CAD build for the part. Positions are in the model's coordinates, mm. Coordinates: 2 decimals unless noted, no trailing zeros. Order: outer loops, then holes, each group sorted by start corner. A loop starts at its lowest first (then second) coordinate and runs counter-clockwise, first axis right, second up. Notation, with made-up numbers: (56.25, 17) - (86.25, 17) arc R18 ccw to (86.25, 40) - close; hole circle Ø1 at (86.5, 40.5). An arc over 180 degrees is marked (long way). Use one line per item in the form item = value.
```python
from build123d import *
from OCP.BRepFilletAPI import BRepFilletAPI_MakeChamfer

# Parameters (mm, degrees)
SKETCH1_W             = 60
SKETCH1_H             = 180
BOSS_EXTRUDE1_DEPTH   = 6
CHAMFER2_SIZE         = 10
BOSS_EXTRUDE3_DEPTH   = 6
BOSS_EXTRUDE4_DEPTH   = 6
CHAMFER14_SIZE        = 2
CHAMFER16_SIZE        = 7
CHAMFER16_SIZE2       = 56.79198309
CHAMFER17_SIZE        = 2
SKETCH59_W            = 21.7
SKETCH59_H            = 5
BOSS_EXTRUDE5_DEPTH   = 6
CHAMFER19_SIZE        = 5
CUT_EXTRUDE28_DEPTH   = 112.04216162
CHAMFER20_SIZE        = 3
CHAMFER20_SIZE2       = 3.484649721
CUT_EXTRUDE29_DEPTH   = 111.166083192
CHAMFER24_SIZE        = 1
CUT_EXTRUDE31_DEPTH   = 111.166083332
SKETCH66_R            = 6
BOSS_EXTRUDE6_DEPTH   = 6
BOSS_EXTRUDE7_DEPTH   = 6
BOSS_EXTRUDE8_DEPTH   = 6
BOSS_EXTRUDE9_DEPTH   = 6
F_3_0MM_DOWEL_HOLE3_D = 3.5


with BuildPart() as part:
    # Sketch1 → Boss-Extrude1 (new body)
    with BuildSketch(Plane(origin=(0, 0, 0), x_dir=(1, 0, 0), z_dir=(0, 1, 0))):
        Rectangle(SKETCH1_W, SKETCH1_H)
    extrude(amount=BOSS_EXTRUDE1_DEPTH)

    # Chamfer2
    chamfer2_edges = [part.edges().sort_by_distance(p)[0] for p in [
        (-30, 3, -90),
        (30, 3, -90),
        (30, 3, 90),
        (-30, 3, 90),
    ]]
    chamfer(chamfer2_edges, length=CHAMFER2_SIZE)

    # Sketch52 → Boss-Extrude3 (add, through all)
    with BuildSketch(Plane(origin=(0, 6, 0), x_dir=(1, 0, 0), z_dir=(0, 1, 0))):
        Polygon((45, 53.067924807), (36.85, 44.173760523), (30, 25.3535402), (30, 79.656998575), (33.429823026, 66.856724783), align=None)
        Polygon((-33.429823026, 66.856724783), (-45, 53.067924807), (-36.85, 44.173760523), (-30, 25.3535402), (-30, 79.656998575), align=None)
    extrude(amount=-BOSS_EXTRUDE3_DEPTH)

    # Sketch53 → Boss-Extrude4 (add, through all)
    with BuildSketch(Plane(origin=(0, 6, 0), x_dir=(1, 0, 0), z_dir=(0, 1, 0))):
        Polygon((30, -65.989627063), (30, -80), (39, -98.344262241), (51.212964584, -83.789417822), align=None)
        Polygon((-51.212964584, -83.789417822), (-30, -65.989627063), (-30, -80), (-39, -98.344262241), align=None)
    extrude(amount=-BOSS_EXTRUDE4_DEPTH)

    # Chamfer14
    chamfer14_edges = [part.edges().sort_by_distance(p)[0] for p in [
        (-45.106482292, 6, 91.066840031),
        (45.106482292, 6, 91.066840031),
    ]]
    chamfer(chamfer14_edges, length=CHAMFER14_SIZE)

    # Chamfer16: one chamfer whose edges measure the first distance from different faces: ONE call of the kernel's chamfer builder (chamfer() names one face for all edges)
    chamfer16_edges_1 = [part.edges().sort_by_distance(p)[0] for p in [
        (-30, 3, 65.989627063),
    ]]
    chamfer16_side_1 = [part.faces().sort_by_distance(p)[0] for p in [
        (-40.483474971, 2.971570606, 74.786307045),
    ]]
    chamfer16_edges_2 = [part.edges().sort_by_distance(p)[0] for p in [
        (30, 3, 65.989627063),
    ]]
    chamfer16_side_2 = [part.faces().sort_by_distance(p)[0] for p in [
        (40.483474971, 2.971570606, 74.786307045),
    ]]
    chamfer16 = BRepFilletAPI_MakeChamfer(part.part.solid().wrapped)
    for e in chamfer16_edges_1:
        chamfer16.Add(CHAMFER16_SIZE, CHAMFER16_SIZE2, e.wrapped, chamfer16_side_1[0].wrapped)  # the first distance lies on this face
    for e in chamfer16_edges_2:
        chamfer16.Add(CHAMFER16_SIZE, CHAMFER16_SIZE2, e.wrapped, chamfer16_side_2[0].wrapped)  # the first distance lies on this face
    add(Compound.cast(chamfer16.Shape()), mode=Mode.REPLACE)

    # Chamfer17
    chamfer17_edges = [part.edges().sort_by_distance(p)[0] for p in [
        (39.214911513, 6, -59.962324795),
        (-39.214911513, 6, -59.962324795),
    ]]
    chamfer(chamfer17_edges, length=CHAMFER17_SIZE)

    # Sketch59 → Boss-Extrude5 (add, through all)
    with BuildSketch(Plane(origin=(0, 6, 0), x_dir=(1, 0, 0), z_dir=(0, 1, 0))):
        with Locations((0, -92.5)):
            Rectangle(SKETCH59_W, SKETCH59_H)
    extrude(amount=-BOSS_EXTRUDE5_DEPTH)

    # Chamfer19
    chamfer19_edges = [part.edges().sort_by_distance(p)[0] for p in [
        (0, 0, 95),
    ]]
    chamfer(chamfer19_edges, length=CHAMFER19_SIZE)

    # Sketch61 → Cut-Extrude28 (cut, through all)
    with BuildSketch(Plane.XZ):
        Polygon((30, -79.656998575), (20, -90), (30, -80), align=None)
        Polygon((-30, -80), (-30, -79.656998575), (-20, -90), align=None)
    extrude(amount=-CUT_EXTRUDE28_DEPTH, mode=Mode.SUBTRACT)

    # Chamfer20: one chamfer whose edges measure the first distance from different faces: ONE call of the kernel's chamfer builder (chamfer() names one face for all edges)
    chamfer20_edges_1 = [part.edges().sort_by_distance(p)[0] for p in [
        (-45, 2, -53.067924807),
    ]]
    chamfer20_side_1 = [part.faces().sort_by_distance(p)[0] for p in [
        (-40.821197815, 2.933105821, -48.507562458),
    ]]
    chamfer20_edges_2 = [part.edges().sort_by_distance(p)[0] for p in [
        (45, 2, -53.067924807),
    ]]
    chamfer20_side_2 = [part.faces().sort_by_distance(p)[0] for p in [
        (39.214911513, 2, -59.962324795),
    ]]
    chamfer20_edges_3 = [part.edges().sort_by_distance(p)[0] for p in [
        (-51.212964584, 2, 83.789417822),
        (51.212964584, 2, 83.789417822),
    ]]
    chamfer20 = BRepFilletAPI_MakeChamfer(part.part.solid().wrapped)
    for e in chamfer20_edges_1:
        chamfer20.Add(CHAMFER20_SIZE, CHAMFER20_SIZE2, e.wrapped, chamfer20_side_1[0].wrapped)  # the first distance lies on this face
    for e in chamfer20_edges_2:
        chamfer20.Add(CHAMFER20_SIZE, CHAMFER20_SIZE2, e.wrapped, chamfer20_side_2[0].wrapped)  # the first distance lies on this face
    for e in chamfer20_edges_3:
        chamfer20.Add(CHAMFER20_SIZE, e.wrapped)
    add(Compound.cast(chamfer20.Shape()), mode=Mode.REPLACE)

    # Sketch62 → Cut-Extrude29 (cut, through all)
    with BuildSketch(Plane(origin=(0, 6, 0), x_dir=(1, 0, 0), z_dir=(0, 1, 0))):
        with BuildLine():
            Line((20, 90), (30, 79.656998575))
            Line((30, 79.656998575), (33.429823026, 66.856724783))
            add(Edge.make_bspline(
                [(33.429823026, 66.856724783), (13.849706238, 74.804707739), (20, 74.573823319), (20, 90)],
                knots=[0, 0, 0, 0, 1, 1, 1, 1], degree=3))
        make_face()
        with BuildLine():
            Line((-30, 79.656998575), (-33.429823026, 66.856724783))
            add(Edge.make_bspline(
                [(-33.429823026, 66.856724783), (-13.849706238, 74.804707739), (-20, 74.573823319), (-20, 90)],
                knots=[0, 0, 0, 0, 1, 1, 1, 1], degree=3))
            Line((-20, 90), (-30, 79.656998575))
        make_face()
    extrude(amount=-CUT_EXTRUDE29_DEPTH, mode=Mode.SUBTRACT)

    # Chamfer24
    chamfer24_edges = [part.edges().sort_by_distance(p)[0] for p in [
        (0, 0, -90),
    ]]
    chamfer(chamfer24_edges, length=CHAMFER24_SIZE)

    # Sketch64 → Cut-Extrude31 (cut, through all)
    with BuildSketch(Plane(origin=(0, 6, 0), x_dir=(1, 0, 0), z_dir=(0, 1, 0))):
        with BuildLine():
            Line((36.85, 44.173760523), (25, 5.3535402))
            add(Edge.make_bspline(
                [(25, 5.3535402), (25, 11.888533403), (26.675205792, 28.424746849), (35.495075594, 42.695120001), (36.85, 44.173760523)],
                knots=[0, 0, 0, 0, 0.750989917, 1, 1, 1, 1], degree=3))
        make_face()
        with BuildLine():
            Line((-36.85, 44.173760523), (-25, 5.3535402))
            add(Edge.make_bspline(
                [(-25, 5.3535402), (-25, 11.888533403), (-26.675205792, 28.424746849), (-35.495075594, 42.695120001), (-36.85, 44.173760523)],
                knots=[0, 0, 0, 0, 0.750989917, 1, 1, 1, 1], degree=3))
        make_face()
    extrude(amount=-CUT_EXTRUDE31_DEPTH, mode=Mode.SUBTRACT)

    # Sketch66 → Boss-Extrude6 (add)
    with BuildSketch(Plane(origin=(0, 6, 0), x_dir=(1, 0, 0), z_dir=(0, 1, 0))):
        with Locations((29.320888862, -18)):
            Circle(SKETCH66_R)
        with BuildLine():
            ThreePointArc((25, -13.837078017), (26.973287097, -12.478336668), (29.320888862, -12))
            Line((29.320888862, -12), (25, -12))
            Line((25, -12), (25, -13.837078017))
        make_face()
        with BuildLine():
            Line((25, -24), (29.320888862, -24))
            ThreePointArc((29.320888862, -24), (26.973287097, -23.521663332), (25, -22.162921983))
            Line((25, -22.162921983), (25, -24))
        make_face()
        with Locations((-29.320888862, -18)):
            Circle(SKETCH66_R)
        with BuildLine():
            Line((-25, -12), (-29.320888862, -12))
            ThreePointArc((-29.320888862, -12), (-26.973287097, -12.478336668), (-25, -13.837078017))
            Line((-25, -13.837078017), (-25, -12))
        make_face()
        with BuildLine():
            ThreePointArc((-25, -22.162921983), (-26.973287097, -23.521663332), (-29.320888862, -24))
            Line((-29.320888862, -24), (-25, -24))
            Line((-25, -24), (-25, -22.162921983))
        make_face()
    extrude(amount=-BOSS_EXTRUDE6_DEPTH)

    # Sketch67 → Boss-Extrude7 (add)
    with BuildSketch(Plane.XZ):
        with BuildLine():
            Line((30, -21.733379998), (30, -31.878802778))
            add(Edge.make_bspline(
                [(30, -31.878802778), (26.006043433, -21.746256389), (25, -11.197434735), (25, -5.3535402)],
                knots=[0.328429926, 0.328429926, 0.328429926, 0.328429926, 1, 1, 1, 1], degree=3))
            Line((25, -5.3535402), (30, -21.733379998))
        make_face()
        with BuildLine():
            Line((-30, -21.733379998), (-30, -31.878802778))
            add(Edge.make_bspline(
                [(-25, -5.3535402), (-25, -11.197434735), (-26.006043433, -21.746256389), (-30, -31.878802778)],
                knots=[0, 0, 0, 0, 0.671570074, 0.671570074, 0.671570074, 0.671570074], degree=3))
            Line((-25, -5.3535402), (-30, -21.733379998))
        make_face()
    extrude(amount=-BOSS_EXTRUDE7_DEPTH)

    # Sketch70 → Boss-Extrude8 (add)
    with BuildSketch(Plane(origin=(0, 6, 0), x_dir=(1, 0, 0), z_dir=(0, 1, 0))):
        Polygon((-35.152040134, -68.085732174), (-36.207663424, -69.695157895), (-42.867802278, -72.070563218), (-51.23722065, -79.093339087), (-48.914831255, -81.861054993), (-35.362311102, -70.489140331), align=None)
        Polygon((-37.956015914, -96.380824876), (-29.919310924, -80), (-22.966994839, -86.952316085), (-25.929369827, -92.160839448), (-35.064832642, -99.826402927), align=None)
        Polygon((35.362311102, -70.489140331), (48.914831255, -81.861054993), (51.23722065, -79.093339087), (42.867802278, -72.070563218), (36.207663424, -69.695157895), (35.152040134, -68.085732174), align=None)
        Polygon((37.956015914, -96.380824876), (29.919310924, -80), (22.966994839, -86.952316085), (25.929369827, -92.160839448), (35.064832642, -99.826402927), align=None)
    extrude(amount=-BOSS_EXTRUDE8_DEPTH)

    # Sketch71 → Boss-Extrude9 (add)
    with BuildSketch(Plane(origin=(0, 6, 0), x_dir=(1, 0, 0), z_dir=(0, 1, 0))):
        Polygon((-38.03670499, -96.380824876), (-37.956015914, -96.380824876), (-29.945868659, -80.054131341), (-30, -80), align=None)
        Polygon((29.945868659, -80.054131341), (37.956015914, -96.380824876), (38.03670499, -96.380824876), (30, -80), align=None)
    extrude(amount=-BOSS_EXTRUDE9_DEPTH)

    # Ø3.0mm Dowel Hole3 (through all)
    with Locations(Plane(origin=(0, 6, 0), x_dir=(1, 0, 0), z_dir=(0, 1, 0))):
        with Locations((20, 64.260302334), (-20, 64.260302334), (-14, -65.321451812), (14, -65.321451812)):
            Hole(F_3_0MM_DOWEL_HOLE3_D / 2)


solid = part.part
```
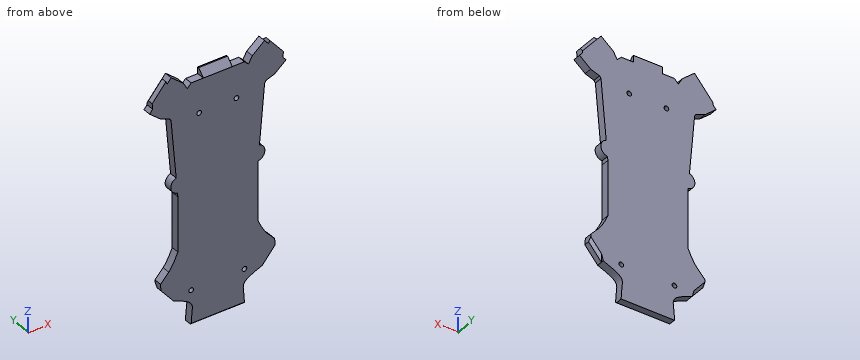
Item 1: Cut at A-A, the plane x = -14. Write the cut outline in (y, z), plus the area to 3 significant figures.
Derived:
outline = (0, -89) - (1, -90) - (6, -90) - (6, 63.57) - (0, 63.57) - close; (0, 67.07) - (6, 67.07) - (6, 90) - (0, 90) - close
area = 1,060 mm²
Item 2: Cut at C-C, the plane y = 3. State how many separate pieces and enclosed holes the cut face has, plus the area to 3 significant figures.
Derived:
separate_pieces = 1
enclosed_holes = 4
area = 12,300 mm²
Item 3: Cut at B-B, the plane z = 18. Write the cut outline in (x, y), plus the area to 3 significant figures.
Derived:
outline = (-35.32, 0) - (35.32, 0) - (35.32, 6) - (-35.32, 6) - close
area = 424 mm²
Item 4: Drop flat-ended pins along their axis: pin 1 (2 mm diameter, centred on y = 2, z = 18, fed in from +X); pin 2 (2.5 mm diameter, centred on y = 3, z = 93.5, fed in from +X); pin 3 (3 mm diameter, centred on x = 14, z = 65.32, fed in from -Y); pin 4 (2.5 mm diameter, centred on y = 4, z = 92.5, fed in from -X). Give the stop position or say it passes through.
Derived:
pin_1 = 35.32
pin_2 = 44.11
pin_3 = through
pin_4 = -44.95
Item 5: Cut at D-D, the plane z = 60.5. Write the cut outline in (x, y).
Derived:
outline = (-34.49, 0) - (34.49, 0) - (34.49, 6) - (-34.49, 6) - close
Item 6: Drill centre lines: line 1 (Z direction, x = -14, y = 3.4); line 2 (X direction, y = 5.75, z = 4.5); line 3 (Z direction, x = -38, y = 1.5). Where is each one in solid material? Low to high. Write a range as [from, to].
Derived:
line_1 = [-90, 63.57], [67.07, 90]
line_2 = [-30, 30]
line_3 = [-61.41, -45.43], [70.33, 96.38]
